Can you work these out from the model? Positions are in its coordinate system, mm. A direction names the side the tool comes from. Give positions to 0.01 mm unless a question says otherwise; leave off trailing zeros. Write each loop counter-clockwise with the first axis right and the second up, starting at its lowest first coordinate (ties: lowest second). Pieces come first, ordered by that corner, then holes.
```python
from build123d import *

# Parameters (mm, degrees)
SKETCH1_R               = 20
BOSS_EXTRUDE1_DEPTH     = 150
BOSS_EXTRUDE2_START     = 40
SKETCH2_R               = 15
BOSS_EXTRUDE2_DEPTH     = 60
SKETCH3_W               = 162.009512726
SKETCH3_H               = 30
CUT_EXTRUDE1_DEPTH      = 405.474968323
CUT_EXTRUDE1_DEPTH_BACK = 405.474968323
SKETCH4_W               = 180
SKETCH4_H               = 153.149018845
CUT_EXTRUDE2_DEPTH      = 405.474968323
CUT_EXTRUDE2_DEPTH_BACK = 405.474968323
CHAMFER1_SIZE           = 4
CHAMFER1_SIZE2          = 21.339042193
CHAMFER1_EDGE_2_SIZE    = 4
CHAMFER1_EDGE_2_SIZE2   = 21.339042193
FILLET1_R               = 4
FILLET2_R               = 8


with BuildPart() as part:
    # Sketch1 → Boss-Extrude1 (new, symmetric)
    with BuildSketch(Plane.XY):
        with BuildLine():
            Line((-195.959179423, 240), (-175.499287748, 240))
            ThreePointArc((-175.499287748, 240), (0, 100), (175.499287748, 240))
            Line((175.499287748, 240), (195.959179423, 240))
            ThreePointArc((195.959179423, 240), (182.049998135, 197.188176092), (158.918539009, 158.571428571))
            Line((158.918539009, 158.571428571), (23.837780851, -18.214285714))
            ThreePointArc((23.837780851, -18.214285714), (0, -30), (-23.837780851, -18.214285714))
            Line((-23.837780851, -18.214285714), (-158.918539009, 158.571428571))
            ThreePointArc((-158.918539009, 158.571428571), (-182.049998135, 197.188176092), (-195.959179423, 240))
        make_face()
        Circle(SKETCH1_R, mode=Mode.SUBTRACT)
    extrude(amount=BOSS_EXTRUDE1_DEPTH, both=True)

    # Sketch2 → Boss-Extrude2 (add)
    with BuildSketch(Plane(origin=(0, 0, 0), x_dir=(1, 0, 0), z_dir=(0, 1, 0)).offset(BOSS_EXTRUDE2_START)):
        with BuildLine():
            Line((-55, -150), (55, -150))
            Line((55, -150), (55, -190))
            Line((55, -190), (31.705882353, -239.823529412))
            ThreePointArc((31.705882353, -239.823529412), (0, -260), (-31.705882353, -239.823529412))
            Line((-31.705882353, -239.823529412), (-55, -190))
            Line((-55, -190), (-55, -150))
        make_face()
        with Locations(Location((0, -225, 0), (0, 0, 270))):
            Circle(SKETCH2_R, mode=Mode.SUBTRACT)
    extrude(amount=BOSS_EXTRUDE2_DEPTH)

    # Sketch3 → Cut-Extrude1 (cut, two sides)
    with BuildSketch(Plane(origin=(0, 0, 0), x_dir=(0, 0, -1), z_dir=(1, 0, 0))) as cut_extrude1_sk:
        with Locations((-231.004756363, 70)):
            Rectangle(SKETCH3_W, SKETCH3_H)
    extrude(amount=CUT_EXTRUDE1_DEPTH, mode=Mode.SUBTRACT)
    extrude(cut_extrude1_sk.sketch, amount=-CUT_EXTRUDE1_DEPTH_BACK, mode=Mode.SUBTRACT)

    # Sketch4 → Cut-Extrude2 (cut, two sides)
    with BuildSketch(Plane(origin=(0, 0, 0), x_dir=(0, 0, -1), z_dir=(1, 0, 0))) as cut_extrude2_sk:
        with Locations((0, 18.425490577)):
            Rectangle(SKETCH4_W, SKETCH4_H)
    extrude(amount=CUT_EXTRUDE2_DEPTH, mode=Mode.SUBTRACT)
    extrude(cut_extrude2_sk.sketch, amount=-CUT_EXTRUDE2_DEPTH_BACK, mode=Mode.SUBTRACT)

    # Chamfer1
    chamfer1_edges = [part.edges().sort_by_distance(p)[0] for p in [
        (110.344044156, 95, 0),
    ]]
    chamfer1_side = [part.faces().sort_by_distance(p)[0] for p in [
        (0, 95, 0),
    ]]
    chamfer(chamfer1_edges, length=CHAMFER1_SIZE, length2=CHAMFER1_SIZE2, reference=chamfer1_side[0])

    # Chamfer1 edge 2
    chamfer1_edge_2_edges = [part.edges().sort_by_distance(p)[0] for p in [
        (-110.344044156, 95, 0),
    ]]
    chamfer1_edge_2_side = [part.faces().sort_by_distance(p)[0] for p in [
        (0, 95, 0),
    ]]
    chamfer(chamfer1_edge_2_edges, length=CHAMFER1_EDGE_2_SIZE, length2=CHAMFER1_EDGE_2_SIZE2, reference=chamfer1_edge_2_side[0])

    # Fillet1
    fillet1_edges = [part.edges().sort_by_distance(p)[0] for p in [
        (0, 95, -90),
        (0, 95, 90),
    ]]
    fillet(fillet1_edges, radius=FILLET1_R)

    # Fillet2
    fillet2_edges = [part.edges().sort_by_distance(p)[0] for p in [
        (-91.37815993, 70.178571429, -150),
        (-182.049998135, 197.188176092, -150),
        (-182.049998135, 197.188176092, 150),
        (-91.37815993, 70.178571429, 150),
        (0, -30, 150),
        (91.37815993, 70.178571429, 150),
        (182.049998135, 197.188176092, 150),
        (182.049998135, 197.188176092, -150),
        (91.37815993, 70.178571429, -150),
        (0, -30, -150),
    ]]
    fillet(fillet2_edges, radius=FILLET2_R)


solid = part.part
```
1) If we mould it in two halves opening along Z, with no side actions, what happens to faces 4 (the face through (115.297, 103.953, 1.26)), 5 (the face through (1, 40, 192)), 6 (the face through (2, 56, 90)), 7 (the face through (43.5, 92.4, 214.6))? For each: +Z half, -Z half, draft (parallel to the pull), parting line (faces both ways), or undercut.
Values follow:
face 4: undercut
face 5: draft
face 6: undercut
face 7: +Z half
2) For faces 1 (the face through (88.52, 70.4, -147.72)), 2 (the face through (-55, 47, 170)), 3 (the face through (55, 47, 170)), which set-ups out of +Z, -Z, +X, -X, +Y, -Y let a thin tool reach every point of the face, with its end or its side?
Values follow:
face 1: -Z, +X, -Y
face 2: +Z, -X, +Y, -Y
face 3: +Z, +X, +Y, -Y
3) Suppose I cut it at A-A on z = -2. Write out the boundary of the cut face in (x, y), plus the area to 3 significant figures.
Values follow:
outline: (-195.96, 240) arc R200 ccw to (-158.92, 158.57) - (-123.3, 111.96) - (-106.34, 95) - (106.34, 95) - (123.3, 111.96) - (158.92, 158.57) arc R200 ccw to (195.96, 240) - (175.5, 240) arc R180 cw to (-175.5, 240) - close
area: 9,940 mm2
4) Suppose I cut it at D-D on y = 0. State how many separate pieces and enclosed holes the cut face has, plus the area to 3 significant figures.
Values follow:
separate pieces: 4
enclosed holes: 0
area: 4,190 mm2
5) For pin 1 Ø16.5 at (y, z) = (94.5, 169) entering from -X; pin 2 Ø16.5 at (y, z) = (44, 170.5) entering from +X; pin 3 Ø10 at (y, z) = (194, 47.5) entering from +X, each with a flat end and sliding along its axis, tell me the tip position at first contact or that it passes through.
Values follow:
pin 1: stops at x = -55
pin 2: stops at x = 55
pin 3: stops at x = 182.86
6) Please list where these lines run through material, in increasing order: L1, parallel to Z at x = 0, y = 48; L2, parallel to Y at x = 1.5, z = 115; L3, parallel to Y at x = -36, z = 157.5.
Values follow:
L1: z = -150 to -90, 90 to 210, 240 to 260
L2: y = -29.96 to -19.94, 19.94 to 100.01
L3: y = 40 to 55, 85 to 100
7) Suppose I cut it at C-C on z = 225. Write out the boundary of the cut face in (x, y), plus the area to 3 significant figures.
Values follow:
outline: (-38.64, 40) - (-15, 40) - (-15, 55) - (-38.64, 55) - close; (-38.64, 85) - (-15, 85) - (-15, 100) - (-38.64, 100) - close; (15, 40) - (38.64, 40) - (38.64, 55) - (15, 55) - close; (15, 85) - (38.64, 85) - (38.64, 100) - (15, 100) - close
area: 1,420 mm2
8) Suppose I cut it at B-B on z = -108.5. Write out the boundary of the cut face in (x, y), plus the area to 3 significant figures.
Values follow:
outline: (-195.96, 240) arc R200 ccw to (-158.92, 158.57) - (-23.84, -18.21) arc R30 ccw to (23.84, -18.21) - (158.92, 158.57) arc R200 ccw to (195.96, 240) - (175.5, 240) arc R180 cw to (-175.5, 240) - close; hole circle Ø40 at (0, 0)
area: 24,300 mm2
